Geometry: final body of the model. Coordinates: model frame, mm. Face numbers are marked on the shaded views. A direction names the side the tool comes from. Give positions to 0.01 mm unless a question says otherwise; leave off trailing zeros. Order: outer loops, then holes, each group sorted by start corner. A loop starts at its lowest first (then second) coordinate and runs counter-clockwise, first axis right, second up. Notation, with made-up numbers: (16.25, 51) - (56.25, 51) arc R9 cw to (56.25, 57) - close; hole circle Ø10 at (46.25, 69.5). An arc over 180 degrees is marked (long way). Write item = value, one per line. Start each with the question number.
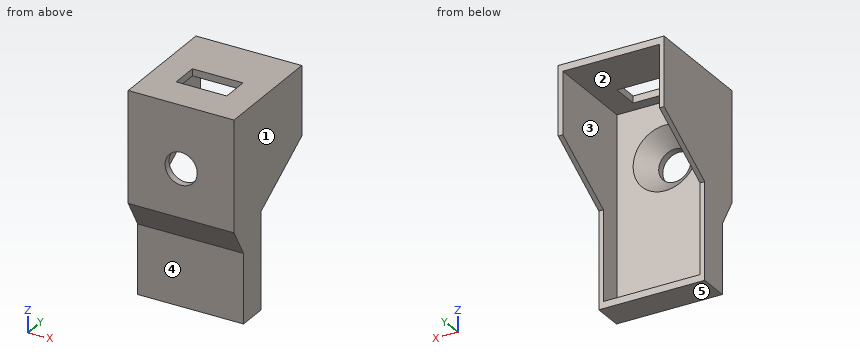
Autodesk Inventor part; units mm, degrees
ref_plane "YZ Plane" through (0, 0, 0) normal (1, 0, 0) x (0, 1, 0)
ref_plane "XZ Plane" through (0, 0, 0) normal (0, 1, 0) x (-1, 0, 0)
ref_plane "XY Plane" through (0, 0, 0) normal (0, 0, 1) x (1, 0, 0)
sketch "Esquisse1" plane through (0, 0, 0) normal (0, 1, 0) x (-1, 0, 0)
  line L0 (-10.5, 21) -> (10.5, 21)
  line L1 (10.5, 21) -> (10.5, -21)
  line L2 (10.5, -21) -> (-10.5, -21)
  line L3 (-10.5, -21) -> (-10.5, 21)
  line L4 (10.5, -21) -> (11.5, -21)
  line L5 (11.5, -21) -> (11.5, 21)
  line L6 (11.5, 21) -> (10.5, 21)
  line L7 (10.5, 21) -> (10.5, -21)
  line L8 (-10.5, 21) -> (-11.5, 21)
  line L9 (-11.5, 21) -> (-11.5, -21)
  line L10 (-11.5, -21) -> (-10.5, -21)
  line L11 (-10.5, -21) -> (-10.5, 21)
  line L12 (11.5, 21) -> (-11.5, 21)
  line L13 (-11.5, 21) -> (-11.5, 22.5)
  line L14 (-11.5, 22.5) -> (11.5, 22.5)
  line L15 (11.5, 22.5) -> (11.5, 21)
  line L16 (11.5, -21) -> (-11.5, -21)
  line L17 (-11.5, -21) -> (-11.5, -22.5)
  line L18 (-11.5, -22.5) -> (11.5, -22.5)
  line L19 (11.5, -22.5) -> (11.5, -21)
  point P0 (0, 0)
  dimension "d0" = 21
  dimension "d1" = 42
  dimension "d2" = 21
  dimension "d3" = 10.5
  dimension "d4" = 1
  dimension "d5" = 1
  dimension "d6" = 1.5
  dimension "d7" = 1.5
extrude "Extrusion1" add sketch "Esquisse1" along normal blind 5
sketch "Esquisse2" plane through (0, 5, 0) normal (0, 1, 0) x (1, 0, 0)
  line L0 (11.5, -22.5) -> (11.5, 22.5)
  line L1 (11.5, 22.5) -> (-11.5, 22.5)
  line L2 (-11.5, 22.5) -> (-11.5, -22.5)
  line L3 (-11.5, -22.5) -> (11.5, -22.5)
  line L4 (-10.5, 21) -> (10.5, 21)
  line L5 (10.5, 21) -> (10.5, -21)
  line L6 (10.5, -21) -> (-10.5, -21)
  line L7 (-10.5, -21) -> (-10.5, 21)
  point P0 (0, 0)
  dimension "d10" = 1
  dimension "d11" = 1
  dimension "d12" = 1.5
  dimension "d13" = 1.5
extrude "Extrusion2" add sketch "Esquisse2" along normal blind 20
sketch "Esquisse3" plane through (0, 5, 0) normal (0, 1, 0) x (1, 0, 0)
  line L0 (10.5, -21) -> (10.5, 21)
  line L1 (-10.5, 21) -> (-10.5, -21)
  line L2 (10.5, -21) -> (0, -21)
  line L3 (0, -21) -> (0, -9) construction
  line L4 (0, -9) -> (10.5, -9) construction
  line L5 (10.5, -9) -> (10.5, -21)
  circle A0 centre (0, -9) radius 3.5
  point P0 (0, 0)
  dimension "d16" = 12
  dimension "d17" = 10.5
  dimension "d18" = 21
  dimension "d19" = 7
extrude "Extrusion3" cut sketch "Esquisse3" against normal through all
sketch "Esquisse4" plane through (-11.5, 0, -22.5) normal (-1, 0, 0) x (0, 0, 1)
  line L0 (45, 0) -> (45, 25)
  line L1 (0, 25) -> (21, 25)
  line L2 (21, 25) -> (21, 10) construction
  line L3 (21, 10) -> (0, 10)
  line L4 (0, 10) -> (0, 25)
  line L5 (45, 25) -> (30, 25)
  line L6 (30, 25) -> (30, 10) construction
  line L7 (30, 10) -> (45, 10) construction
  line L8 (45, 10) -> (45, 25)
  line L9 (21, 10) -> (30, 25)
  line L10 (30, 25) -> (21, 25)
  point P0 (22.5, 0)
  dimension "d22" = 15
  dimension "d23" = 24
  dimension "d24" = 15
extrude "Extrusion4" cut sketch "Esquisse4" against normal through all
sketch "Esquisse5" plane through (-11.5, 0, -22.5) normal (-1, 0, 0) x (0, 0, 1)
  line L0 (0, 0) -> (45, 0)
  line L1 (45, 0) -> (45, 25)
  line L2 (0, 0) -> (15, 0)
  line L3 (15, 0) -> (15, 3.5) construction
  line L4 (15, 3.5) -> (0, 3.5)
  line L5 (0, 3.5) -> (0, 0)
  line L6 (45, 0) -> (21, 0)
  line L7 (21, 0) -> (21, 3.5) construction
  line L8 (21, 3.5) -> (45, 3.5) construction
  line L9 (45, 3.5) -> (45, 0)
  line L10 (15, 3.5) -> (21, 0)
  line L11 (15, 0) -> (21, 0)
  point P0 (22.5, 0)
  dimension "d27" = 3.5
  dimension "d28" = 30
  dimension "d29" = 24
extrude "Extrusion5" cut sketch "Esquisse5" against normal through all
chamfer "Chanfrein1" distance 3.5 angle 45 1 edges at (-3.5, 5, 9)
sketch "Esquisse8" plane through (10.5, 5, 21) normal (0, 0, -1) x (-1, 0, 0)
  line L0 (21, 0) -> (0, 0)
  line L1 (21, 0) -> (21, 20)
  line L2 (0, 0) -> (0, 20)
  line L3 (5, 8.5) -> (16, 8.5)
  line L4 (16, 8.5) -> (16, 2.5)
  line L5 (16, 2.5) -> (5, 2.5)
  line L6 (5, 2.5) -> (5, 8.5)
  point P0 (10.5, -5)
  dimension "d38" = 2.5
  dimension "d39" = 6
  dimension "d40" = 11
  dimension "d41" = 21
  dimension "d42" = 5
extrude "Extrusion6" cut sketch "Esquisse8" against normal through all
equation "\"d5\" = d4"
equation "\"d7\" = d6"
equation "\"d11\" = d10"
equation "\"d13\" = d12"
equation "\"d17\" = 0.5 * d18"
equation "\"d42\" = -0.5 * d40 + 0.5 * d41"
properties part number "anti_axe_2"
Q1. Section D-D, the plane y = 23.5. Return the cut outline in (x, z).
Q2. Section B-B, the plane x = 0. Return the cut outline in (y, z), then the cut area to 3 significant figures.
Q3. Section C-C, the plane z = 9. Return the cut outline in (x, y).
Q4. Material intervals for line 1 along X through (y, z) = (20.5, 8); line 2 along X through (y, z) = (0.6, 9); line 3 along Z through (x, y) = (7.25, 8.25), sorted ascending. Write a range as from..to.
Q5. Contact query for flat-ended pins moving along their axis: pin 1 (11 mm diameter, centred on x = 0, z = 9, fed in from +Y); pin 2 (12 mm diameter, centred on x = -0.5, z = -18.5, fed in from -Y); pin 3 (10.5 mm diameter, centred on x = 2.5, z = -8, fed in from +Y). Output: stop coordinate, or through.
Q6. Section A-A, the plane y = 11.5. Return the cut outline in (x, z), then the cut area to 3 significant figures.
Q7. Set-up query: the marked faces 1 and 2. Return all of +Z, -Z, +X, -X, +Y, -Y with unobstructed straight access to the full face (end or side cutting, diameter ignored); none if empty.
Q8. Pull-direction query (Z, two-part tool) for the marked faces 3, 4 and 5; classes: +Z half, -Z half, draft (parallel to the pull), parting line (faces both ways), or undercut.
The answers:
q1.outline = (-11.5, 6.6) - (-10.5, 6.6) - (-10.5, 21) - (10.5, 21) - (10.5, 6.6) - (11.5, 6.6) - (11.5, 22.5) - (-11.5, 22.5) - close
q2.outline = (0, -1.5) - (3.5, -7.5) - (3.5, -22.5) - (10, -22.5) - (10, -21) - (5, -21) - (5, 2) - (1.5, 5.5) - (0, 5.5) - close; (0, 12.5) - (1.5, 12.5) - (5, 16) - (5, 21) - (7.5, 21) - (7.5, 22.5) - (0, 22.5) - close; (13.5, 21) - (25, 21) - (25, 22.5) - (13.5, 22.5) - close
q2.area = 143 mm²
q3.outline = (-11.5, 0) - (-3.5, 0) - (-3.5, 1.5) - (-7, 5) - (-10.5, 5) - (-10.5, 25) - (-11.5, 25) - close; (3.5, 0) - (11.5, 0) - (11.5, 25) - (10.5, 25) - (10.5, 5) - (7, 5) - (3.5, 1.5) - close
q4.line_1 = -11.5..-10.5, 10.5..11.5
q4.line_2 = -11.5..-3.5, 3.5..11.5
q4.line_3 = -22.5..-21, 21..22.5
q5.pin_1 = 3.5
q5.pin_2 = 3.5
q5.pin_3 = 5
q6.outline = (-11.5, -0.6) - (-10.5, -0.6) - (-10.5, 21) - (-5.5, 21) - (-5.5, 22.5) - (-11.5, 22.5) - close; (5.5, 21) - (10.5, 21) - (10.5, -0.6) - (11.5, -0.6) - (11.5, 22.5) - (5.5, 22.5) - close
q6.area = 61.2 mm²
q7.face_1 = +Z, -Z, +X, +Y, -Y
q7.face_2 = +Y
q8.face_3 = undercut
q8.face_4 = draft
q8.face_5 = -Z half
